```python
from build123d import *

# Parameters (mm, degrees)
F0_W     = 33
F0_H     = 22
F0_R     = 5
F1_DEPTH = 2


with BuildPart() as f1:
    # F0 (on Top) → F1 (new body)
    with BuildSketch(Plane.XY):
        Polygon((0, 70), (0, 0), (140, 0), (140, 70), (140, 85), (125, 85), (125, 70), (15, 70), (15, 85), (0, 85), align=None)
        with Locations((25, 20)):
            Rectangle(F0_W, F0_H, mode=Mode.SUBTRACT)
        with Locations((70, 20)):
            Rectangle(F0_W, F0_H, mode=Mode.SUBTRACT)
        with Locations((115, 20)):
            Rectangle(F0_W, F0_H, mode=Mode.SUBTRACT)
        with Locations((25, 50)):
            Rectangle(F0_W, F0_H, mode=Mode.SUBTRACT)
        with Locations((7.5, 77.5)):
            Circle(F0_R, mode=Mode.SUBTRACT)
        with Locations((70, 50)):
            Rectangle(F0_W, F0_H, mode=Mode.SUBTRACT)
        with Locations((115, 50)):
            Rectangle(F0_W, F0_H, mode=Mode.SUBTRACT)
        with Locations((132.5, 77.5)):
            Circle(F0_R, mode=Mode.SUBTRACT)
    extrude(amount=F1_DEPTH)


solid = f1.part
```
Can you work these out from the model? Positions are in its coordinate system, mm. Coordinates: 2 decimals unless noted, no trailing zeros. Order: outer loops, then holes, each group sorted by start corner. A loop starts at its lowest first (then second) coordinate and runs counter-clockwise, first axis right, second up.
1. If we section it at D-D (y = 77.5): Please give me the cut outline in (x, z), then the cut area to 3 significant figures.
2. If we section it at C-C (z = 0.6): Give the number of separate pieces and of enclosed holes in the cut face, then the cut area to 3 significant figures.
3. Thinking about a two-plate mould opening in Y: for faces 1 (the face through (6.42, 72.62, 0.99)), 2 (the face through (53, 34, 2)), which applies, +Y half, -Y half, draft (parallel to the pull), parting line (faces both ways), or undercut?
4. I need wall thicknesses on line 1 (Y direction, x = 19, z = 1.15); line 2 (X direction, y = 13, z = 1.4); line 3 (Y direction, x = 130, z = 1.35). Which ranges of each line are inside material? Lowest first, please.
5. I'm going to push flat-ended pins straight in: pin 1 (1 mm diameter, centred on y = 20, z = 1.5, fed in from -X); pin 2 (0.6 mm diameter, centred on x = 71.5, z = 1, fed in from +Y). Where does each tip first touch, or does it pass through?
6. If we section it at B-B (x = 77): Please give me the cut outline in (y, z).
7. If we section it at A-A (y = 45): Please give me the cut outline in (x, z), then the cut area to 3 significant figures.
Entries:
1. outline: (0, 0) - (2.5, 0) - (2.5, 2) - (0, 2) - close; (12.5, 0) - (15, 0) - (15, 2) - (12.5, 2) - close; (125, 0) - (127.5, 0) - (127.5, 2) - (125, 2) - close; (137.5, 0) - (140, 0) - (140, 2) - (137.5, 2) - close
1. area: 20.0 mm2
2. separate pieces: 1
2. enclosed holes: 8
2. area: 5,740 mm2
3. face 1: undercut
3. face 2: draft
4. line 1: y = 0 to 9, 31 to 39, 61 to 70
4. line 2: x = 0 to 8.5, 41.5 to 53.5, 86.5 to 98.5, 131.5 to 140
4. line 3: y = 0 to 9, 31 to 39, 61 to 73.17, 81.83 to 85
5. pin 1: stops at x = 0
5. pin 2: stops at y = 70
6. outline: (0, 0) - (9, 0) - (9, 2) - (0, 2) - close; (31, 0) - (39, 0) - (39, 2) - (31, 2) - close; (61, 0) - (70, 0) - (70, 2) - (61, 2) - close
7. outline: (0, 0) - (8.5, 0) - (8.5, 2) - (0, 2) - close; (41.5, 0) - (53.5, 0) - (53.5, 2) - (41.5, 2) - close; (86.5, 0) - (98.5, 0) - (98.5, 2) - (86.5, 2) - close; (131.5, 0) - (140, 0) - (140, 2) - (131.5, 2) - close
7. area: 82.0 mm2
